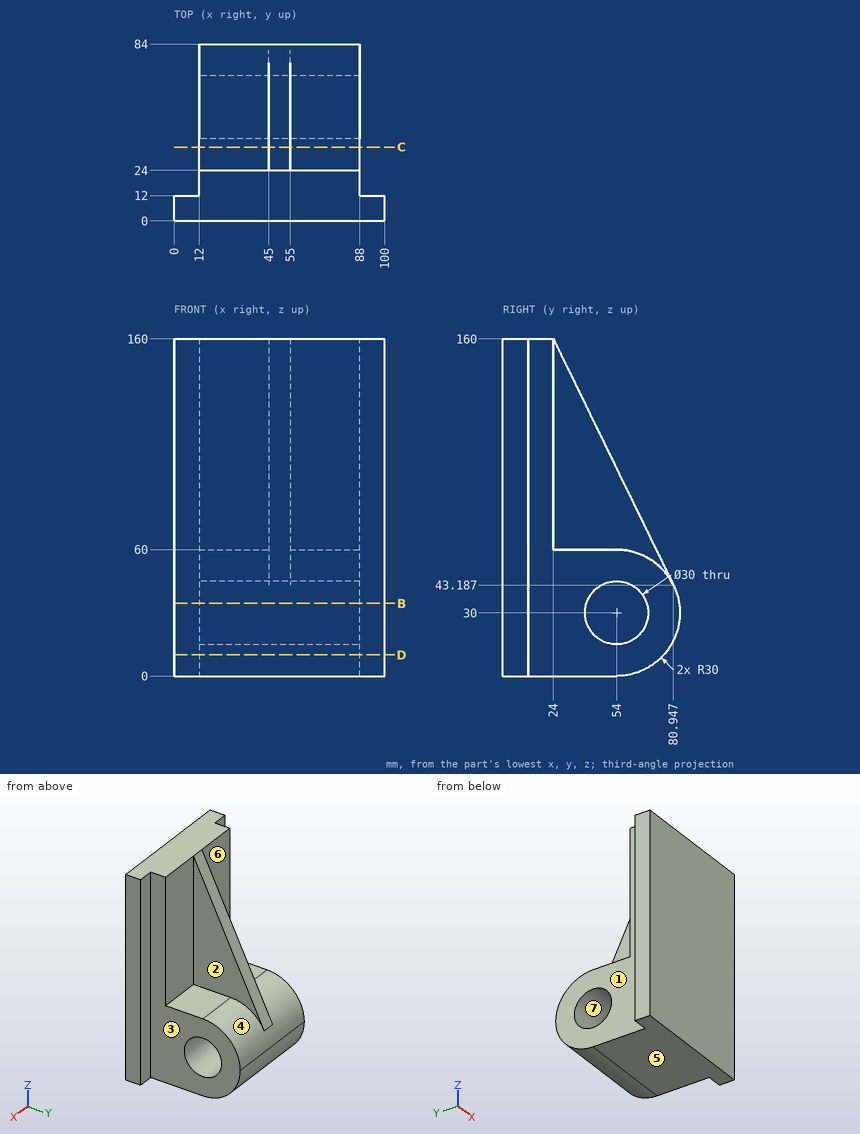
Here's the drawing with two shaded views (mm, measured from the low corner). I have some questions. A direction names the side the tool comes from. Round coordinates to 2 decimals unless told otherwise and drop trailing zeros. Write each loop counter-clockwise with the first axis right and the second up, starting at its lowest first coordinate (ties: lowest second). Pieces come first, ordered by that corner, then holes. Notation, with made-up numbers: M 13,43.5 L 35,43.5 A18 ccw 35,69.5 Z; hole C -34.5,-38.5 d7. An arc over 180 degrees is marked long. Write each question's results on one line, items separated by ' | '. Start each with the question number.
1. Imagine slicing it at C-C on y = 35. List the corners of the cut face in (x, z) for me (1 decimal), and give its area (3 significant figures).
2. I need wall thicknesses on L1, parallel to Y at x = 69, z = 30; L2, parallel to X at y = 54, z = 75; L3, parallel to Y at x = 4.5, z = 66. Which ranges of each line are inside material? Lowest first, please. Write a range as from..to.
3. On a 3-axis mill with a long thin cutter (end or side, diameter ignored), from which of +Z, -Z, +X, -X, +Y, -Y can I reach the whole of each face in a straight line? I mean the marked faces 1, 2 and 3. Say none if no direction works.
4. Imagine slicing it at B-B on z = 34.5. List the corners of the cut face in (x, y) for me.
5. Imagine slicing it at D-D on z = 10. List the corners of the cut face in (x, y) for me.
6. I'm going to push flat-ended pins straight in: pin 1 Ø2 at (x, z) = (85.5, 45) entering from -Y; pin 2 Ø1.5 at (y, z) = (32, 77.5) entering from -X; pin 3 Ø6 at (x, z) = (3.5, 91) entering from +Y; pin 4 Ø2 at (x, z) = (74.5, 69.5) entering from +Y. Where does each tip first touch, or does it pass through?
7. Thinking about a two-plate mould opening in Z: for the marked faces 4, 5, 6 and 7, which applies, +Z half, -Z half, draft (parallel to the pull), parting line (faces both ways), or undercut?
Result sheet:
1) outline: M 12,0 L 88,0 L 88,60 L 55,60 L 55,137.4 L 45,137.4 L 45,60 L 12,60 Z | area: 5,330 mm^2
2) L1: y = 0..39, 69..84 | L2: x = 45..55 | L3: y = 0..12
3) face 1: +Z, -Z, -X, +Y | face 2: +Z, +X, +Y | face 3: +Z, -Z, +X, +Y
4) outline: M 0,0 L 100,0 L 100,12 L 88,12 L 88,39.69 L 12,39.69 L 12,12 L 0,12 Z; M 12,68.31 L 88,68.31 L 88,83.66 L 12,83.66 Z
5) outline: M 0,0 L 100,0 L 100,12 L 88,12 L 88,76.36 L 12,76.36 L 12,12 L 0,12 Z
6) pin 1: stops at y = 0 | pin 2: stops at x = 45 | pin 3: stops at y = 12 | pin 4: stops at y = 24
7) face 4: +Z half | face 5: -Z half | face 6: draft | face 7: undercut
